For this review, take the finished solid that the model builds, in its own axes (mm). A direction names the side the tool comes from. Coordinates: 2 decimals unless noted, no trailing zeros. Answer as a JSON object with one key per item and string values. Group by question number.
1) Draft analysis for pull direction X (two halves, no side actions). For faces 1 (the flat face through (12, -6, 5)), 2 (the cylindrical face through (23, 1, 1)), 3 (the flat face through (12, -2, 3)), 4 (the cylindrical face through (2, 1, 1)), state which applies: +X half, -X half, draft (parallel to the pull), parting line (faces both ways), or undercut.
2) For pin 1 (4 mm diameter, centred on x = 22.5, y = 5.5, fed in from -Z); pin 2 (2 mm diameter, centred on y = 0, z = 4, fed in from -X); pin 3 (3 mm diameter, centred on y = -1.5, z = 1, fed in from +X), all flat-tipped, find the tip position at first contact; note any pin that passes through.
3) Wall thickness on L1, parallel to X at y = -6, z = 3.8; L2, parallel to Y at x = 12.5, z = 4.6: over which ranges is each line inside the solid? List them lowest first.
4) Machinability: for faces 5 (the cylindrical face through (11.741, -9.417, 3.986)), 6 (the cylindrical face through (12.395, 11.641, 1.426)), which of the approach directions +Z, -Z, +X, -X, +Y, -Y give a long, thin tool a straight path to every point of the face, cutting with its end or side? Answer none if there is none.
from build123d import *

# Parameters (mm, degrees)
F0_W     = 25
F0_H     = 25
F1_DEPTH = 5
F2_R     = 5
F3_R     = 4.99999
F5_START = 3
F4_R     = 3.5
F5_DEPTH = 22


# Not quite as in the source:
# - a fillet or chamfer is up to 0.001 mm smaller than in the source, because OpenCascade refuses the exact size


with BuildPart() as f1:
    # F0 (on Top) → F1 (new body)
    with BuildSketch(Plane.XY):
        with Locations((12.5, 0.6441110272)):
            Rectangle(F0_W, F0_H)
    extrude(amount=F1_DEPTH)

    # F2
    f2_edges = [f1.edges().sort_by_distance(p)[0] for p in [
        (0, 13.144111, 2.5),
        (25, 13.144111, 2.5),
        (0, -11.855889, 2.5),
        (25, -11.855889, 2.5),
    ]]
    fillet(f2_edges, radius=F2_R)

    # F3 (radius 5 in the source; OpenCascade refuses exactly that, so slightly less here)
    f3_edges = [f1.edges().sort_by_distance(p)[0] for p in [
        (12.5, -11.855889, 0),
        (0, 0.644111, 0),
        (25, 0.644111, 0),
        (12.5, 13.144111, 0),
    ]]
    fillet(f3_edges, radius=F3_R)

    # F4 (on Top) → F5 (cut)
    with BuildSketch(Plane.XY.offset(F5_START)):
        with BuildLine():
            ThreePointArc((19.5, -6), (9.1718039657, 0.1581743364), (8.6648253836, -11.8558889728))
            Line((8.6648253836, -11.8558889728), (16.3351746164, -11.8558889728))
            ThreePointArc((16.3351746164, -11.8558889728), (18.6581743364, -9.3281960343), (19.5, -6))
        make_face()
        with Locations((12.5, -6)):
            Circle(F4_R, mode=Mode.SUBTRACT)
    extrude(amount=F5_DEPTH, mode=Mode.SUBTRACT)


solid = f1.part
Output values:
{
 "1": {"face 1": "draft", "face 2": "+X half", "face 3": "undercut", "face 4": "-X half"},
 "2": {"pin 1": "stops at z = 0.03", "pin 2": "stops at x = 0", "pin 3": "stops at x = 24.33"},
 "3": {"L1": "x = 0.15 to 5.5, 9 to 16, 19.5 to 24.85", "L2": "y = -9.5 to -2.5, 1 to 13.13"},
 "4": {"face 5": "+Z", "face 6": "-Z, +X, -X, +Y"}
}
